Print and shaded views of the part. All mm, measured from the part's lowest x, y and z. A direction names the side the tool comes from. Round coordinates to 2 decimals unless told otherwise and drop trailing zeros. Write each loop counter-clockwise with the first axis right and the second up, starting at its lowest first coordinate (ties: lowest second). Pieces come first, ordered by that corner, then holes. Notation, with made-up numbers: (33.5, 87) - (56.5, 87) arc R26 ccw to (56.5, 113) - close; hole circle Ø5 at (67.5, 8.5). An arc over 180 degrees is marked (long way). Put each result on its own line as item: value. Start each with the question number.
Item 1: Mould opens along Y. For the marked faces 1, 2 and 3 say: released by +Y, released by -Y, zero draft, split by the parting line, or undercut.
Item 2: 3-axis set-ups, long thin cutter, end or side, ignore diameter. For the marked faces 4 and 5: which of +Z, -Z, +X, -X, +Y, -Y reach the whole face in a straight line?
Item 3: Cut at B-B (y = 6.5). Give the cut face in (x, z).
Item 4: Cut at C-C (z = 4). Give the cut face in (x, y), and give its area (3 significant figures).
Item 5: Cut at D-D (z = 0.5). Give the cut face in (x, y), and give its area (3 significant figures).
Item 6: Cut at A-A (x = 5). Give the cut face in (y, z).
Item 7: Pin check, flat tip, straight feed: pin 1 Ø5.5 at (x, y) = (15, 6.5) entering from -Z. Stop position of the tip, or through.
Item 8: Drill centre lines: line 1 (X direction, y = 6.5, z = 6.25); line 2 (Y direction, x = 25, z = 6.25); line 3 (Z direction, x = 15, y = 1.8). Where is each one in solid material? Low to high. Write a range as from..to.
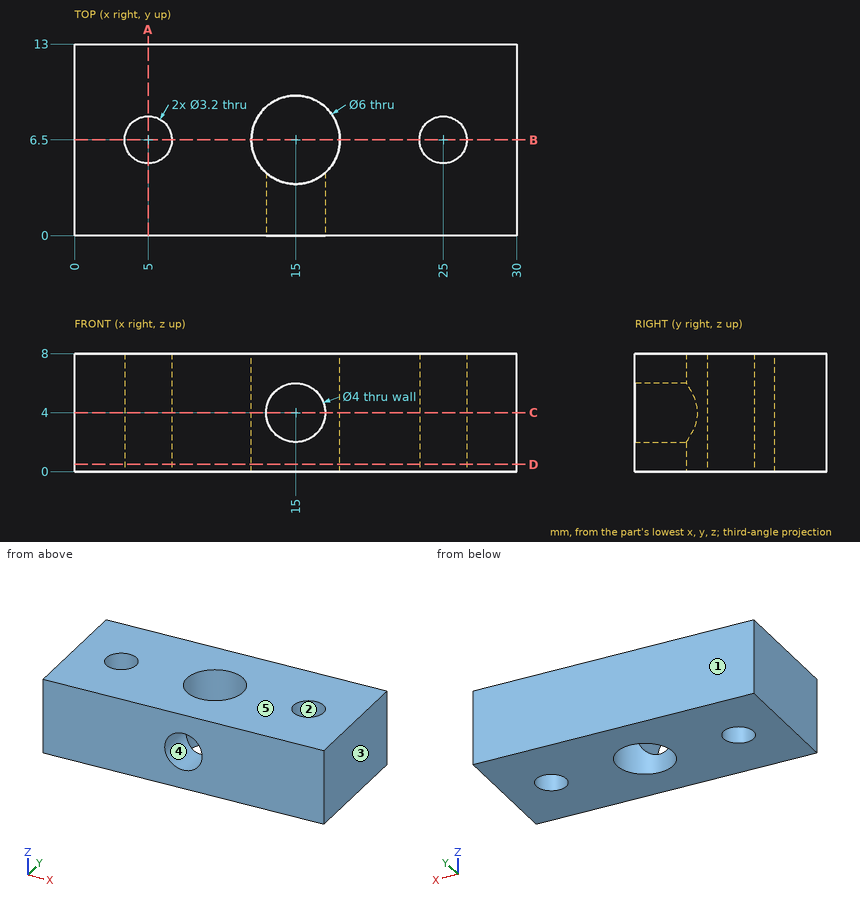
Output values:
1. face 1: released by +Y
1. face 2: undercut
1. face 3: zero draft
2. face 4: -Y
2. face 5: +Z, +X, -X, +Y, -Y
3. outline: (0, 0) - (3.4, 0) - (3.4, 8) - (0, 8) - close; (6.6, 0) - (12, 0) - (12, 8) - (6.6, 8) - close; (18, 0) - (23.4, 0) - (23.4, 8) - (18, 8) - close; (26.6, 0) - (30, 0) - (30, 8) - (26.6, 8) - close
4. outline: (0, 0) - (13, 0) - (13, 4.26) arc R3 cw (long way) to (17, 4.26) - (17, 0) - (30, 0) - (30, 13) - (0, 13) - close; hole circle Ø3.2 at (5, 6.5); hole circle Ø3.2 at (25, 6.5)
4. area: 331 mm2
5. outline: (0, 0) - (30, 0) - (30, 13) - (0, 13) - close; hole circle Ø3.2 at (5, 6.5); hole circle Ø6 at (15, 6.5); hole circle Ø3.2 at (25, 6.5)
5. area: 346 mm2
6. outline: (0, 0) - (4.9, 0) - (4.9, 8) - (0, 8) - close; (8.1, 0) - (13, 0) - (13, 8) - (8.1, 8) - close
7. pin 1: through
8. line 1: 0..3.4, 6.6..12, 18..23.4, 26.6..30
8. line 2: 0..4.9, 8.1..13
8. line 3: 0..2, 6..8
